from build123d import *

# Parameters (mm, degrees)
BOSS_EXTRUDE3_DEPTH      = 10
M3_CLEARANCE_HOLE1_D     = 3.6
M3_CLEARANCE_HOLE1_DEPTH = 5
M3_CLEARANCE_HOLE1_TIP   = 1.081549114


with BuildPart() as part:
    # Sketch3 → Boss-Extrude3 (new body)
    with BuildSketch(Plane.XY):
        with BuildLine():
            ThreePointArc((10.627637959, -5.374147741), (8.187588203, -0.208463055), (4.251688797, 3.93241088))
            ThreePointArc((4.251688797, 3.93241088), (2.191837366, 4.729023368), (0, 5))
            ThreePointArc((0, 5), (-3.823420235, 3.222026956), (-4.927665225, -0.847416917))
            ThreePointArc((-4.927665225, -0.847416917), (0.77252532, -5.462986054), (7.504596942, -8.374147741))
            ThreePointArc((7.504596942, -8.374147741), (9.507210052, -7.33333117), (10.627637959, -5.374147741))
        make_face()
    extrude(amount=BOSS_EXTRUDE3_DEPTH)

    # M3 Clearance Hole1
    with Locations(Plane.XY.offset(10)):
        with Locations((0, 2)):
            Hole(M3_CLEARANCE_HOLE1_D / 2, depth=M3_CLEARANCE_HOLE1_DEPTH)
            with Locations((0, 0, -(M3_CLEARANCE_HOLE1_DEPTH + M3_CLEARANCE_HOLE1_TIP / 2))):  # 118° drill point
                Cone(0, M3_CLEARANCE_HOLE1_D / 2, M3_CLEARANCE_HOLE1_TIP, mode=Mode.SUBTRACT)


solid = part.part
Check sheet for the modelled part. Datum: model origin and axes. Units: mm. A direction names the side the tool comes from. Round coordinates to 2 decimals unless told otherwise and drop trailing zeros. Loops run counter-clockwise (first coordinate to the right, second up) from the corner with the lowest first, then second, coordinate; pieces in that order, holes last. Notation, with made-up numbers: (48, -37) - (59, -37) arc R3 cw to (59, -33) - close; hole circle Ø9 at (46.25, 84.5). An arc over 180 degrees is marked (long way). Answer as CSV lines item,"result". Start each with the question number.
Item 1: Set-up check for faces 4 (the cylindrical face through (9.48, -7.36, 4.93)), 5 (the cylindrical face through (0.234, 3.785, 7.465)): record each of +Z, -Z, +X, -X, +Y, -Y from which the full face is reachable in a straight line by a thin tool's end or side.
Item 2: Section check A-A (z = 7). Record the boundary of the cut face in (x, y).
Item 3: Section check B-B (z = 2.5). Record the boundary of the cut face in (x, y).
Item 4: Scan lines: line 1 (Y direction, x = -1.5, z = 6); line 2 (X direction, y = 2, z = 7.4); line 3 (Y direction, x = -0.25, z = 8.5). Record each from-to range of solid material in increasing order. Write a range as [from, to].
Item 5: Depth check by flat-ended pin: P1, Ø4, axis at y = 3.5, z = 6.5, coming from the +X side; P2, Ø4, axis at x = 9, z = 8.5, coming from the +Y side; P3, Ø4, axis at x = 2, z = 6, coming from the -Y side. Enter the tip coordinate at first touch or a pass-through.
Item 6: Section check D-D (x = 2.5). Record the boundary of the cut face in (y, z), and give its area (3 significant figures).
Item 7: Section check C-C (y = -5). Record the boundary of the cut face in (x, z).
Item 8: Release check for a two-part mould opening along Y. For faces 1 (the cylindrical face through (2.22, 4.72, 4.93)), 2 (the conical face through (-0.07, 1.69, 4.11)), 3 (the flat face through (3, -2, 10)) record: +Y half, -Y half, draft (parallel to the pull), parting line (faces both ways), or undercut.
Report:
1,face 4,"+Z, -Z, +X, -Y"
1,face 5,"+Z"
2,outline,"(-4.93, -0.85) arc R27 ccw to (7.5, -8.37) arc R4 ccw to (10.63, -5.37) arc R18 ccw to (4.25, 3.93) arc R9 ccw to (0, 5) arc R5 ccw to start; hole circle Ø3.6 at (0, 2)"
3,outline,"(-4.93, -0.85) arc R27 ccw to (7.5, -8.37) arc R4 ccw to (10.63, -5.37) arc R18 ccw to (4.25, 3.93) arc R9 ccw to (0, 5) arc R5 ccw to start"
4,line 1,"y = [-3.92, 1.01], [2.99, 4.77]"
4,line 2,"x = [-4.58, -1.8], [1.8, 6.4]"
4,line 3,"y = [-4.81, 0.22], [3.78, 4.99]"
5,P1,"stops at x = 6.86"
5,P2,"stops at y = 1.34"
5,P3,"stops at y = -7.13"
6,outline,"(-6.42, 0) - (4.65, 0) - (4.65, 10) - (-6.42, 10) - close"
6,area,"111 mm2"
7,outline,"(0.03, 0) - (10.51, 0) - (10.51, 10) - (0.03, 10) - close"
8,face 1,"+Y half"
8,face 2,"undercut"
8,face 3,"draft"
